The drawing under review shows one solid part. Ordinate dimensions are in mm from its lowest x, y, z. A direction names the side the tool comes from. Coordinates: 2 decimals unless noted, no trailing zeros. Order: outer loops, then holes, each group sorted by start corner. A loop starts at its lowest first (then second) coordinate and runs counter-clockwise, first axis right, second up.
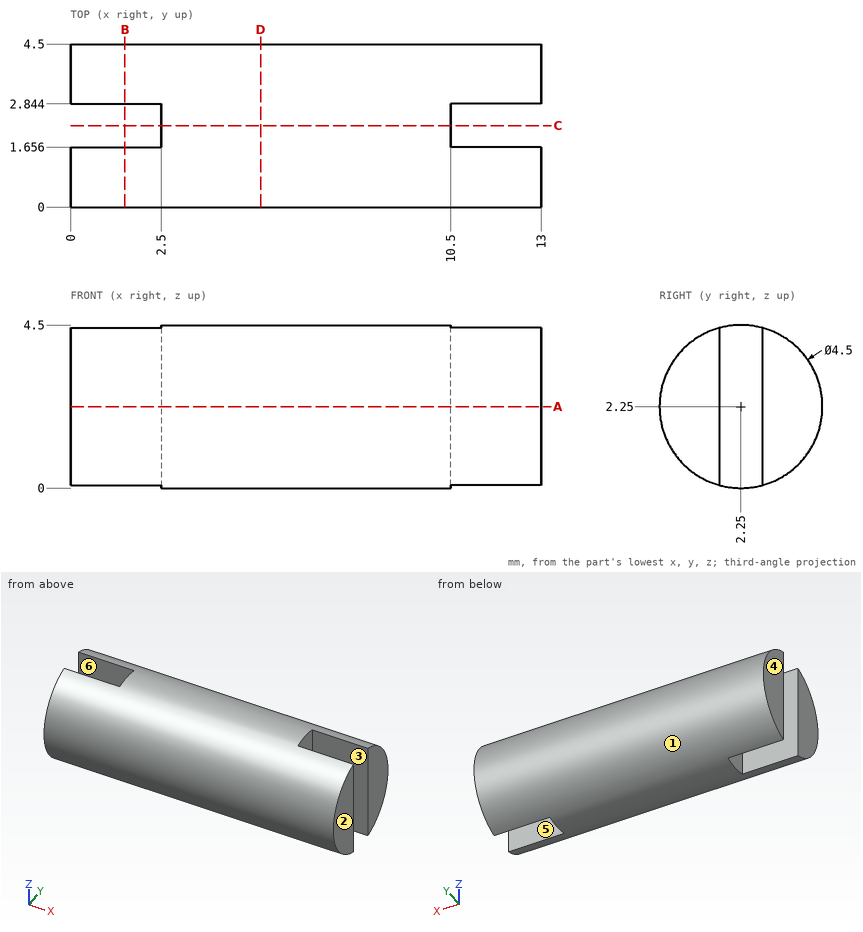
(1) We need section D-D, the plane x = 5.25. Write out the cut boundary in (y, z), and give its area (3 significant figures).
A:
outline: circle Ø4.5 at (2.25, 2.25)
area: 15.9 mm2
(2) We need section B-B, the plane x = 1.5. Write out the cut boundary in (y, z), and give its area (3 significant figures).
A:
outline: (1.66, 0.08) - (1.66, 4.42) arc R2.25 ccw to start; (2.84, 0.08) arc R2.25 ccw to (2.84, 4.42) - close
area: 10.6 mm2
(3) Wall thickness on probe 1 along X at (y, z) = (2.5, 2.6); probe 2 along Y at (x, z) = (11, 3.5); probe 3 along Y at (x, z) = (2, 4.05): over which ranges is each line inside the solid? List them lowest first.
A:
probe 1: x = 2.5 to 10.5
probe 2: y = 0.38 to 1.66, 2.84 to 4.12
probe 3: y = 0.9 to 1.66, 2.84 to 3.6
(4) Machinability: for the marked faces 4, 5 and 6, which of the approach directions +Z, -Z, +X, -X, +Y, -Y give a long, thin tool a straight path to every point of the face, cutting with its end or side? Answer none if there is none.
A:
face 4: +Z, -Z, -X, +Y, -Y
face 5: +Z, -Z, +X
face 6: +Z, -Z, -X
(5) Draft analysis for pull direction Y (two halves, no side actions). For the marked faces 1, 2 and 3, state which applies: released by +Y, released by -Y, zero draft, split by the parting line, or undercut.
A:
face 1: split by the parting line
face 2: zero draft
face 3: undercut
(6) We need section C-C, the plane y = 2.25. Write out the cut boundary in (x, z).
A:
outline: (2.5, 0) - (10.5, 0) - (10.5, 4.5) - (2.5, 4.5) - close
(7) For pin 1 Ø0.6 at (y, z) = (2.5, 2) entering from +X; pin 2 Ø2 at (x, z) = (11.5, 1.5) entering from +Y; pin 3 Ø1 at (x, z) = (3.5, 0.5) entering from +Y; pin 4 Ø1.2 at (x, z) = (1, 1.5) entering from -Y (3 decimals), all flat-tipped, find the tip position at first contact; note any pin that passes through.
A:
pin 1: stops at x = 10.5
pin 2: stops at y = 4.5
pin 3: stops at y = 4.12
pin 4: stops at y = 0.005
(8) We need section A-A, the plane z = 2.25. Write out the cut boundary in (x, y).
A:
outline: (0, 0) - (13, 0) - (13, 1.66) - (10.5, 1.66) - (10.5, 2.84) - (13, 2.84) - (13, 4.5) - (0, 4.5) - (0, 2.84) - (2.5, 2.84) - (2.5, 1.66) - (0, 1.66) - close
